Part model, mm, in its own coordinate system. A direction names the side the tool comes from. Round coordinates to 2 decimals unless told otherwise and drop trailing zeros. Loops run counter-clockwise (first coordinate to the right, second up) from the corner with the lowest first, then second, coordinate; pieces in that order, holes last.
1) Band-saw the part on B-B, the plane z = 2.05. Write the cut outline in (x, y).
2) Mould opens along X. For faces 4 (the cylindrical face through (-3.35, 25.82, 1.99)), 5 (the flat face through (-19, 63, 1)), 6 (the flat face through (-12, 50, 1)) say: +X half, -X half, draft (parallel to the pull), parting line (faces both ways), or undercut.
3) Drop flat-ended pins along their axis: P1, Ø1.5, axis at y = 43.5, z = 1.5, coming from the -X side; P2, Ø2, axis at x = -14, y = 17.5, coming from the -Z side; P3, Ø1, axis at y = 20.5, z = 1.5, coming from the +X side. Give the stop position or say it passes through.
4) Probe line 1 (X direction, y = 60.5, z = 0.5); line 2 (X direction, y = 45, z = 0.6); line 3 (X direction, y = 3, z = 1.45). List the from-to ranges inside material, lowest first.
5) Band-saw the part on A-A, the plane x = -15. Write the cut outline in (y, z), then the cut area to 3 significant figures.
6) Band-saw the part on D-D, the plane y = 21.5. Write the cut outline in (x, z), then the cut area to 3 significant figures.
7) 3-axis set-ups, long thin cutter, end or side, ignore diameter. For faces 1 (the cylindrical face through (-5.306, 32.597, 1.479)), 2 (the cylindrical face through (-31.52, 2.85, 1.99)), 3 (the flat face through (-27, 42, 1)): which of +Z, -Z, +X, -X, +Y, -Y reach the whole face in a straight line?
8) Band-saw the part on C-C, the plane x = -24. Write the cut outline in (y, z), then the cut area to 3 significant figures.
from build123d import *

# Parameters (mm, degrees)
RESSALTO_EXTRUS_O2_DEPTH                  = 3
BROCA_DE_ROSQUEAR_PARA_TARRAXA_DE_M2_51_D = 2.05
FURO_DE_DI_METRO_6_0_6_2_D                = 6
FURO_DE_DI_METRO_6_0_6_2_DEPTH            = 2
FURO_DE_DI_METRO_6_0_6_2_TIP              = 1.802581857
ESCAREADO_PARA_SFHCS_M31_AT_2_COUNT       = 2
ESCAREADO_PARA_SFHCS_M31_AT_2_PITCH       = 9
FILETE1_R                                 = 5


with BuildPart() as part:
    # Esboço1 → Ressalto-extrusão2 (new body)
    with BuildSketch(Plane.XY):
        with BuildLine():
            Line((-12, 30.768414179), (-12, 63))
            Line((-12, 63), (-27, 63))
            Line((-27, 63), (-27, 19.018288858))
            ThreePointArc((-27, 19.018288858), (-30.719082421, 12.125728279), (-32.710572622, 4.551236075))
            ThreePointArc((-32.710572622, 4.551236075), (-29.299973416, 0.038164719), (-24.786902061, 3.448763925))
            ThreePointArc((-24.786902061, 3.448763925), (-17.695825587, 17.695825587), (-3.448763925, 24.786902061))
            ThreePointArc((-3.448763925, 24.786902061), (-0.038164719, 29.299973416), (-4.551236075, 32.710572622))
            ThreePointArc((-4.551236075, 32.710572622), (-8.332397539, 31.957259931), (-12, 30.768414179))
        make_face()
    extrude(amount=RESSALTO_EXTRUS_O2_DEPTH)

    # Broca de rosquear para tarraxa de M2.51 (through all)
    with Locations(Plane.XY.offset(3)):
        with Locations((-28.748737342, 4), (-4, 28.748737342)):
            Hole(BROCA_DE_ROSQUEAR_PARA_TARRAXA_DE_M2_51_D / 2)

    # Furo de diâmetro Ø6.0 (6)2
    with Locations(Plane.XY.offset(3)):
        with Locations((-28.748737342, 4), (-4, 28.748737342)):
            Hole(FURO_DE_DI_METRO_6_0_6_2_D / 2, depth=FURO_DE_DI_METRO_6_0_6_2_DEPTH)
            with Locations((0, 0, -(FURO_DE_DI_METRO_6_0_6_2_DEPTH + FURO_DE_DI_METRO_6_0_6_2_TIP / 2))):  # 118° drill point
                Cone(0, FURO_DE_DI_METRO_6_0_6_2_D / 2, FURO_DE_DI_METRO_6_0_6_2_TIP, mode=Mode.SUBTRACT)

    # Esboço13 → Escareado para SFHCS M31 (revolve, cut)
    with BuildSketch(Plane(origin=(-24, 60.5, 3), x_dir=(0, -1, 0), z_dir=(1, 0, 0))):
        Polygon((0, 0), (0, 3), (1.7, 3), (1.7, 1.66), (3.36, 0), align=None)
    escareado_para_sfhcs_m31 = revolve(axis=Axis((-24, 60.5, 9.35), (0, 0, -1)), mode=Mode.SUBTRACT)

    # Escareado para SFHCS M31 at 2: Escareado para SFHCS M31 ×2
    with Locations(*[(i * ESCAREADO_PARA_SFHCS_M31_AT_2_PITCH, 0, 0) for i in range(1, ESCAREADO_PARA_SFHCS_M31_AT_2_COUNT)]):
        add(escareado_para_sfhcs_m31, mode=Mode.SUBTRACT)

    # Filete1
    filete1_edges = [part.edges().sort_by_distance(p)[0] for p in [
        (-27, 19.018288858, 1.5),
        (-12, 30.768414179, 1.5),
    ]]
    fillet(filete1_edges, radius=FILETE1_R)


solid = part.part
Reported:
1. outline: (-32.71, 4.55) arc R4 ccw to (-24.79, 3.45) arc R25.03 cw to (-3.45, 24.79) arc R4 ccw to (-4.55, 32.71) arc R33.03 ccw to (-6.08, 32.46) arc R5 cw to (-12, 37.38) - (-12, 63) - (-27, 63) - (-27, 20.54) arc R5 cw to (-27.79, 17.84) arc R33.03 ccw to start; hole circle Ø6 at (-28.75, 4); hole circle Ø4.82 at (-24, 60.5); hole circle Ø4.82 at (-15, 60.5); hole circle Ø6 at (-4, 28.75)
2. face 4: undercut
2. face 5: draft
2. face 6: +X half
3. P1: stops at x = -27
3. P2: passes through
3. P3: stops at x = -13.61
4. line 1: x = -27 to -25.7, -22.3 to -16.7, -13.3 to -12
4. line 2: x = -27 to -12
4. line 3: x = -32.62 to -31.58, -25.92 to -24.88
5. outline: (20.03, 0) - (58.8, 0) - (58.8, 1.34) - (57.14, 3) - (20.03, 3) - close; (62.2, 0) - (63, 0) - (63, 2.14) - (62.2, 1.34) - close
5. area: 116 mm2
6. outline: (-27, 0) - (-12.81, 0) - (-12.81, 3) - (-27, 3) - close
6. area: 42.6 mm2
7. face 1: +Z, -Z, +Y
7. face 2: +Z
7. face 3: +Z, -Z, -X, +Y
8. outline: (7.09, 0) - (58.8, 0) - (58.8, 1.34) - (57.14, 3) - (7.09, 3) - close; (62.2, 0) - (63, 0) - (63, 2.14) - (62.2, 1.34) - close
8. area: 155 mm2
